For this review, take the finished solid that the model builds, in its own axes (mm). Face numbers are marked on the shaded views. Give positions to 0.01 mm unless a question says otherwise; leave off trailing zeros. Loops run counter-clockwise (first coordinate to the right, second up) from the corner with the lowest first, then second, coordinate; pieces in that order, holes last. Notation, with made-up numbers: (-15.5, 8.25) -> (-1.5, 8.25) arc R29 cw to (-1.5, 33.25) -> close; hole circle Ø6 at (67.5, 61.5). An arc over 180 degrees is marked (long way). Write each question's results on one line, items separated by ' | '. Start each with the question number.
```python
from build123d import *

# Parameters (mm, degrees)
SKETCH1_R           = 20
BOSS_EXTRUDE1_DEPTH = 68
SKETCH2_R           = 4
CUT_EXTRUDE1_DEPTH  = 10
SKETCH3_R           = 2.5
BOSS_EXTRUDE2_DEPTH = 27
CUT_EXTRUDE2_DEPTH  = 6
CHAMFER1_SIZE       = 3
CUT_EXTRUDE3_START  = -12
SKETCH5_R           = 20
SKETCH5_R_2         = 19
CUT_EXTRUDE3_DEPTH  = 2
LPATTERN1_COUNT     = 15
LPATTERN1_PITCH     = 3


with BuildPart() as part:
    # Sketch1 → Boss-Extrude1 (new body)
    with BuildSketch(Plane.XY):
        Circle(SKETCH1_R)
    extrude(amount=BOSS_EXTRUDE1_DEPTH)

    # Sketch2 → Cut-Extrude1 (cut)
    with BuildSketch(Plane.XY.offset(68)):
        Circle(SKETCH2_R)
    extrude(amount=-CUT_EXTRUDE1_DEPTH, mode=Mode.SUBTRACT)

    # Sketch3 → Boss-Extrude2 (add)
    with BuildSketch(Plane.XY.offset(58)):
        Circle(SKETCH3_R)
    extrude(amount=BOSS_EXTRUDE2_DEPTH)

    # Sketch4 → Cut-Extrude2 (cut)
    with BuildSketch(Plane.XY.offset(85)):
        Polygon((-73.022353661, 2), (-1.5, 2), (1.5, 2), (73.022353661, 2), (73.022353661, 145.044707322), (-73.022353661, 145.044707322), align=None)
    extrude(amount=-CUT_EXTRUDE2_DEPTH, mode=Mode.SUBTRACT)

    # Chamfer1
    chamfer1_edges = [part.edges().sort_by_distance(p)[0] for p in [
        (-20, 0, 0),
        (-20, 0, 68),
    ]]
    chamfer(chamfer1_edges, length=CHAMFER1_SIZE)

    # Sketch5 → Cut-Extrude3 (cut)
    with BuildSketch(Plane.XY.offset(68).offset(CUT_EXTRUDE3_START)):
        Circle(SKETCH5_R)
        Circle(SKETCH5_R_2, mode=Mode.SUBTRACT)
    cut_extrude3 = extrude(amount=-CUT_EXTRUDE3_DEPTH, mode=Mode.SUBTRACT)

    # LPattern1: Cut-Extrude3 ×15
    with Locations(*[(0, 0, -i * LPATTERN1_PITCH) for i in range(1, LPATTERN1_COUNT)]):
        add(cut_extrude3, mode=Mode.SUBTRACT)


solid = part.part
```
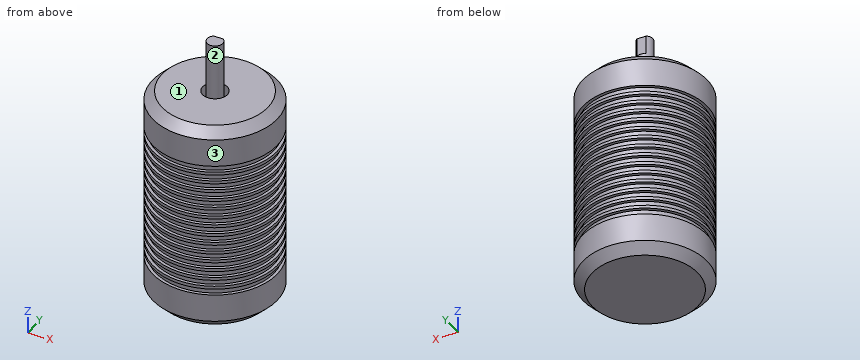
1. Draft analysis for pull direction X (two halves, no side actions). For the marked faces 1, 2 and 3, state which applies: released by +X, released by -X, zero draft, split by the parting line, or undercut.
2. For pin 1 Ø4 at (y, z) = (9, 11) entering from +X (3 decimals); pin 2 Ø5 at (x, z) = (-11.5, 11) entering from +Y; pin 3 Ø12 at (x, y) = (-6, 8) entering from +Z, all flat-tipped, find the tip position at first contact; note any pin that passes through.
3. Wall thickness on L1, parallel to Y at x = 0, z = 66; L2, parallel to Y at x = 0, z = 62; L3, parallel to Z at x = 7, y = -7: over which ranges is each line inside the solid? List them lowest first.
4. We need section A-A (z = 67). Write out the cut boundary in (x, y).
Response:
1) face 1: zero draft | face 2: undercut | face 3: split by the parting line
2) pin 1: stops at x = 18.735 | pin 2: stops at y = 17.86 | pin 3: stops at z = 68
3) L1: y = -19 to -4, -2.5 to 2.5, 4 to 19 | L2: y = -20 to -4, -2.5 to 2.5, 4 to 20 | L3: z = 0 to 68
4) outline: circle Ø36 at (0, 0); circle Ø5 at (0, 0); hole circle Ø8 at (0, 0)
